Read the model definition and answer for the solid it produces. Units are mm, in the model's axes. A direction names the side the tool comes from. Coordinates: 2 decimals unless noted, no trailing zeros. Order: outer loops, then holes, each group sorted by start corner. A loop starts at its lowest first (then second) coordinate and runs counter-clockwise, first axis right, second up. Notation, with made-up numbers: (52.25, -14.5) -> (106.25, -14.5) arc R28 cw to (106.25, 9.5) -> close; hole circle Ø7 at (1.5, 82). An arc over 180 degrees is marked (long way). Use CSV: the item, a comma, the result in double quotes.
```python
from build123d import *

# Parameters (mm, degrees)
BOSS_EXTRUDE1_DEPTH      = 20
BOSS_EXTRUDE1_DEPTH_BACK = 20
CUT_EXTRUDE1_REACH       = 75.759
SKETCH3_W                = 34
SKETCH3_H                = 25.2
CUT_EXTRUDE2_DEPTH       = 3
CUT_EXTRUDE3_REACH       = 57.409


with BuildPart() as part:
    # Sketch1 → Boss-Extrude1 (new, two sides: drawn at the far end of the back side and taken through both)
    with BuildSketch(Plane.XY.offset(-BOSS_EXTRUDE1_DEPTH_BACK)):
        Polygon((-20, -4.8), (41.191180555, -4.8), (16.16, -36), (-20, -36), align=None)
    extrude(amount=BOSS_EXTRUDE1_DEPTH + BOSS_EXTRUDE1_DEPTH_BACK)

    # Cut-Extrude1: up to this plane
    cut_extrude1_end = Plane(origin=(38.851180555, -2.922661458, -20), z_dir=(0.7799999999999999, -0.6257795138864808, 0))
    # Sketch3 → Cut-Extrude1 (cut, up to the surface)
    with BuildSketch(Plane.ZY.offset(20), mode=Mode.PRIVATE) as cut_extrude1_sk1:
        with Locations((0, -20.4)):
            Rectangle(SKETCH3_W, SKETCH3_H)
    cut_extrude1_tool1 = split(extrude(cut_extrude1_sk1.sketch, amount=-CUT_EXTRUDE1_REACH, mode=Mode.PRIVATE), bisect_by=cut_extrude1_end, keep=Keep.BOTH, mode=Mode.PRIVATE)
    add(cut_extrude1_tool1.solids().sort_by_distance((-20, -20.4, 0))[0], mode=Mode.SUBTRACT)

    # Sketch4 → Cut-Extrude2 (cut)
    with BuildSketch(Plane(origin=(25.06363275, -20.108087075, 0), x_dir=(0, 0, 1), z_dir=(-0.78, 0.6257795138864807, 0))):
        with BuildLine():
            Line((-17, 9.329856704), (-17, -5.264662815))
            ThreePointArc((-17, -5.264662815), (0, -16.467403056), (17, -5.264662815))
            Line((17, -5.264662815), (17, 9.329856704))
            ThreePointArc((17, 9.329856704), (15.039919545, 12.805285563), (12.38022373, 15.779598814))
            Line((12.38022373, 15.779598814), (-12.38022373, 15.779598814))
            ThreePointArc((-12.38022373, 15.779598814), (-15.039919545, 12.805285563), (-17, 9.329856704))
        make_face()
    extrude(amount=-CUT_EXTRUDE2_DEPTH, mode=Mode.SUBTRACT)

    # Sketch5 → Cut-Extrude3 (cut, up to next)
    with BuildSketch(Plane(origin=(0, -4.8, 0), x_dir=(1, 0, 0), z_dir=(0, 1, 0)), mode=Mode.PRIVATE) as cut_extrude3_sk1:
        with BuildLine():
            Line((0, 6.25), (-20, 6.25))
            Line((-20, 6.25), (-20, -6.25))
            Line((-20, -6.25), (0, -6.25))
            ThreePointArc((0, -6.25), (6.25, 0), (0, 6.25))
        make_face()
    cut_extrude3_tool1 = extrude(cut_extrude3_sk1.sketch, amount=-CUT_EXTRUDE3_REACH, mode=Mode.PRIVATE) & part.part
    add(cut_extrude3_tool1.solids().sort_by_distance((-7.506569, -4.8, 0))[0], mode=Mode.SUBTRACT)


solid = part.part
```
Item 1: A tool of negligible diameter and unlimited length cuts with its end or side. For faces 1 (the flat face through (-10, -6, -6.25)), 2 (the flat face through (14.835, -32.858, -4.958)), 3 (the flat face through (36.092, -8.726, 0.173)), from which of +Z, -Z, +X, -X, +Y, -Y can it reach the whole face along a straight path? Write none if from no direction.
Return value:
face 1,"-X, +Y"
face 2,"-X"
face 3,"-X, -Y"
Item 2: Find section A-A, the plane z = 5. Give the vertices of the cut face in (x, y).
Return value:
outline,"(-20, -36) -> (16.16, -36) -> (17.53, -34.29) -> (15.19, -32.42) -> (14.72, -33) -> (-20, -33) -> close; (3.75, -7.8) -> (34.94, -7.8) -> (37.28, -9.68) -> (41.19, -4.8) -> (3.75, -4.8) -> close"
Item 3: Find section C-C, the plane x = -4. Give the vertices of the cut face in (y, z).
Return value:
outline,"(-36, -20) -> (-4.8, -20) -> (-4.8, -6.25) -> (-7.8, -6.25) -> (-7.8, -17) -> (-33, -17) -> (-33, 17) -> (-7.8, 17) -> (-7.8, 6.25) -> (-4.8, 6.25) -> (-4.8, 20) -> (-36, 20) -> close"
Item 4: Find section B-B, the plane y = -17. Give the vertices of the cut face in (x, z).
Return value:
outline,"(-20, -20) -> (31.4, -20) -> (31.4, -17) -> (-20, -17) -> close; (-20, 17) -> (31.4, 17) -> (31.4, 20) -> (-20, 20) -> close"
Item 5: The mould has two halves that part along Y. Classify faces 4 (the flat face through (-3, -33, 0)), 5 (the flat face through (-2, -36, 0)), 6 (the flat face through (4, -20, 20)): +Y half, -Y half, draft (parallel to the pull), parting line (faces both ways), or undercut.
Return value:
face 4,"undercut"
face 5,"-Y half"
face 6,"draft"
Item 6: Straight lines are drawn through the part: line 1 along Z through (x, y) = (-11.5, -24.5); line 2 along Y through (x, z) = (5.5, -16); line 3 along Y through (x, z) = (15.5, -11). For each, find the intervals that lie inside material, in ascending order.
Return value:
line 1,"z = -20 to -17, 17 to 20"
line 2,"y = -36 to -33, -7.8 to -4.8"
line 3,"y = -36 to -32.03, -7.8 to -4.8"
Item 7: Find section D-D, the plane z = 14. Give the vertices of the cut face in (x, y), then the cut area to 3 significant figures.
Return value:
outline,"(-20, -36) -> (16.16, -36) -> (21.11, -29.83) -> (18.77, -27.96) -> (14.72, -33) -> (-20, -33) -> close; (-20, -7.8) -> (34.94, -7.8) -> (33.9, -9.09) -> (36.24, -10.97) -> (41.19, -4.8) -> (-20, -4.8) -> close"
area,"316 mm^2"
